```python
from build123d import *

# Parameters (mm, degrees)
SKETCH3_W           = 210
SKETCH3_H           = 50
BOSS_EXTRUDE1_DEPTH = 5
SKETCH8_R           = 1.5
BOSS_EXTRUDE2_DEPTH = 7.62


with BuildPart() as part:
    # Sketch3 → Boss-Extrude1 (new body)
    with BuildSketch(Plane.XY):
        Polygon((-265, -25), (-105, -25), (-105, 25), (-265, 15), align=None)
        with BuildLine():
            Line((-275, -25), (-265, -25))
            Line((-265, -25), (-265, 15))
            ThreePointArc((-265, 15), (-284.634416342, -1.341395914), (-275, -25))
        make_face()
        Rectangle(SKETCH3_W, SKETCH3_H)
        Polygon((105, 25), (105, -25), (265, -25), (265, 15), align=None)
        with BuildLine():
            Line((265, 15), (265, -25))
            Line((265, -25), (275, -25))
            ThreePointArc((275, -25), (284.634416342, -1.341395914), (265, 15))
        make_face()
    extrude(amount=BOSS_EXTRUDE1_DEPTH)

    # Sketch8 → Boss-Extrude2 (add)
    with BuildSketch(Plane.XY.offset(5)):
        with Locations((0, 11)):
            Circle(SKETCH8_R)
        with Locations((0, 1)):
            Circle(SKETCH8_R)
        with Locations((0, -9)):
            Circle(SKETCH8_R)
        with Locations((0, -19)):
            Circle(SKETCH8_R)
        with Locations((50.8, 11)):
            Circle(SKETCH8_R)
        with Locations((50.8, -9)):
            Circle(SKETCH8_R)
        with Locations((50.8, 1)):
            Circle(SKETCH8_R)
        with Locations((50.8, -19)):
            Circle(SKETCH8_R)
        with Locations((101.6, 11)):
            Circle(SKETCH8_R)
        with Locations((101.6, -9)):
            Circle(SKETCH8_R)
        with Locations((101.6, 1)):
            Circle(SKETCH8_R)
        with Locations((101.6, -19)):
            Circle(SKETCH8_R)
        with Locations((-50.8, 11)):
            Circle(SKETCH8_R)
        with Locations((-50.8, 1)):
            Circle(SKETCH8_R)
        with Locations((-50.8, -9)):
            Circle(SKETCH8_R)
        with Locations((-50.8, -19)):
            Circle(SKETCH8_R)
        with Locations((-101.6, 11)):
            Circle(SKETCH8_R)
        with Locations((-101.6, 1)):
            Circle(SKETCH8_R)
        with Locations((-101.6, -9)):
            Circle(SKETCH8_R)
        with Locations((-101.6, -19)):
            Circle(SKETCH8_R)
    extrude(amount=BOSS_EXTRUDE2_DEPTH)


solid = part.part
```
The listing builds one solid part. Answer for the finished solid, in the listing's coordinates (mm). Coordinates: 2 decimals unless noted, no trailing zeros. Loops run counter-clockwise (first coordinate to the right, second up) from the corner with the lowest first, then second, coordinate; pieces in that order, holes last. Notation, with made-up numbers: (15, 56.25) -> (41, 56.25) arc R21 cw to (41, 65.25) -> close; hole circle Ø5 at (37.5, 9). An arc over 180 degrees is marked (long way). Use one line per item in the form item = value. Start each with the question number.
Item 1: The part is cut by section A-A on x = -74. Determine the outline of the cut face in (y, z).
Item 2: Consider L1, parallel to X at y = -18.5, z = 8.5; L2, parallel to Z at x = -207.5, y = -18; L3, parallel to Y at x = 217.5, z = 3. Determine where each line is inside the solid, lowest interval first. Write a range as [from, to].
Item 3: Flat-ended cylindrical pins translate along their axes: pin 1 Ø5 at (x, y) = (5.5, 7.5) entering from +Z; pin 2 Ø3 at (y, z) = (7.5, 2.5) entering from -X; pin 3 Ø6 at (y, z) = (-3, 2) entering from -X. Find the tip coordinate at first contact, or state that the pin passes through.
Item 4: The mould has two halves that part along Y. Classify faces 1 (the face through (-4, 0, 0)), 2 (the face through (186.12, 19.93, 2.46)), 3 (the face through (-284.54, -0.97, 2.46)): released by +Y, released by -Y, zero draft, split by the parting line, or undercut.
Answer key:
q1.outline = (-25, 0) -> (25, 0) -> (25, 5) -> (-25, 5) -> close
q2.L1 = [-103.01, -100.19], [-52.21, -49.39], [-1.41, 1.41], [49.39, 52.21], [100.19, 103.01]
q2.L2 = [0, 5]
q2.L3 = [-25, 17.97]
q3.pin_1 = 5
q3.pin_2 = -281.24
q3.pin_3 = -285.27
q4.face_1 = zero draft
q4.face_2 = released by +Y
q4.face_3 = split by the parting line
